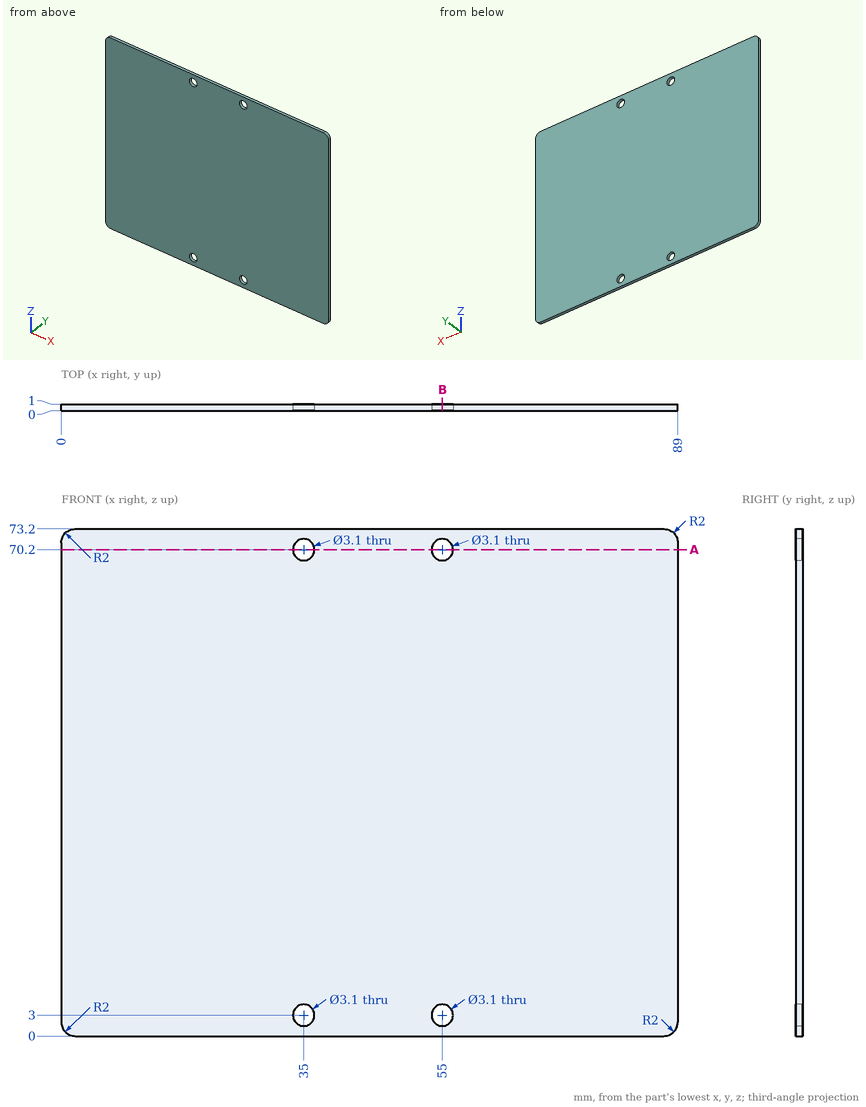
Part print with two shaded views. Sizes in mm from the minimum x, y, z corner. Coordinates: 2 decimals unless noted, no trailing zeros. Write each loop counter-clockwise with the first axis right and the second up, starting at its lowest first coordinate (ties: lowest second). Pieces come first, ordered by that corner, then holes. Notation, with made-up numbers: (61, -2) -> (72, -2) arc R17 cw to (72, 21) -> close; hole circle Ø2 at (-6.5, -34). An arc over 180 degrees is marked (long way). Return JSON: item names as keys, results as strings. Group by question number.
Q1. Cut at A-A, the plane z = 70.2. Give the cut face in (x, y), then the cut area to 3 significant figures.
Q2. Cut at B-B, the plane x = 55. Give the cut face in (y, z).
Q3. Drill centre line: line 1 (X direction, y = 0.5, z = 3). Where is it in solid material? Low to high.
Q4. Flat gauge pin, fed straight in: pin 1 (1.9 mm diameter, centred on x = 35, z = 70.2, fed in from +Y). Where does the tip first touch, or does it go through?
Returned:
{
 "1": {"outline": "(0, 0) -> (33.45, 0) -> (33.45, 1) -> (0, 1) -> close; (36.55, 0) -> (53.45, 0) -> (53.45, 1) -> (36.55, 1) -> close; (56.55, 0) -> (89, 0) -> (89, 1) -> (56.55, 1) -> close", "area": "82.8 mm2"},
 "2": {"outline": "(0, 0) -> (1, 0) -> (1, 1.45) -> (0, 1.45) -> close; (0, 4.55) -> (1, 4.55) -> (1, 68.65) -> (0, 68.65) -> close; (0, 71.75) -> (1, 71.75) -> (1, 73.2) -> (0, 73.2) -> close"},
 "3": {"line 1": "x = 0 to 33.45, 36.55 to 53.45, 56.55 to 89"},
 "4": {"pin 1": "passes through"}
}
